```python
from build123d import *

# Parameters (mm, degrees)
SKETCH1_W           = 100
SKETCH1_H           = 6
BOSS_EXTRUDE1_DEPTH = 5
SKETCH2_W           = 100
SKETCH2_H           = 4.1675
CUT_EXTRUDE1_DEPTH  = 4
CUT_EXTRUDE2_DEPTH  = 20


with BuildPart() as part:
    # Sketch1 → Boss-Extrude1 (new body)
    with BuildSketch(Plane(origin=(0, 0, 0), x_dir=(1, 0, 0), z_dir=(0, 1, 0))):
        Rectangle(SKETCH1_W, SKETCH1_H)
    extrude(amount=BOSS_EXTRUDE1_DEPTH)

    # Sketch2 → Cut-Extrude1 (cut)
    with BuildSketch(Plane(origin=(0, 5, 0), x_dir=(1, 0, 0), z_dir=(0, 1, 0))):
        Rectangle(SKETCH2_W, SKETCH2_H)
    extrude(amount=-CUT_EXTRUDE1_DEPTH, mode=Mode.SUBTRACT)

    # Sketch3 → Cut-Extrude2 (cut)
    with BuildSketch(Plane.XY.offset(3)):
        Polygon((50, 0), (41.339745962, 5), (50, 5), align=None)
    extrude(amount=-CUT_EXTRUDE2_DEPTH, mode=Mode.SUBTRACT)


solid = part.part
```
Geometry check sheet. Reference: the model listing, model coordinates, mm. A direction names the side the tool comes from. Round coordinates to 2 decimals unless told otherwise and drop trailing zeros. Loops run counter-clockwise (first coordinate to the right, second up) from the corner with the lowest first, then second, coordinate; pieces in that order, holes last. Notation, with made-up numbers: (82, 55) - (119, 55) arc R14 ccw to (119, 73) - close; hole circle Ø10 at (11.25, 29.5). An arc over 180 degrees is marked (long way). Write item = value, one per line. Start each with the question number.
1. Thickness scan on line 1 (Z direction, x = -28, y = 2.5); line 2 (Y direction, x = -38, z = -0.1); line 3 (X direction, y = 0.5, z = -1.65). Record the ranges inside material, lowest first.
2. Section check C-C on z = -0.15. Enter the section's corners in (x, y), then the cut area to 3 significant figures.
3. Section check B-B on x = 33. Enter the section's corners in (y, z), then the cut area to 3 significant figures.
4. Set-up check for faces 1 (the face through (-2, 1, 0)), 2 (the face through (48.617, 0.798, 0.042)): record each of +Z, -Z, +X, -X, +Y, -Y from which the full face is reachable in a straight line by a thin tool's end or side.
5. Depth check by flat-ended pin: pin 1 (1 mm diameter, centred on y = 3.5, z = 1, fed in from +X); pin 2 (3 mm diameter, centred on x = 11, z = 0.5, fed in from +Y); pin 3 (3 mm diameter, centred on y = 4, z = -2, fed in from +X). Enter the tip coordinate at first touch or a pass-through.
6. Mould release check, pull along Z, two halves, no side actions. Record for faces 3 (the face through (-1, 2, 3)), 4 (the face through (-1, 2, -3)), 5 (the face through (-2, 3, 2.084)): released by +Z, released by -Z, zero draft, split by the parting line, or undercut.
7. Section check A-A on y = 3.25. Enter the section's corners in (x, z).
Working result:
q1.line_1 = -3 to -2.08, 2.08 to 3
q1.line_2 = 0 to 1
q1.line_3 = -50 to 49.13
q2.outline = (-50, 0) - (50, 0) - (48.27, 1) - (-50, 1) - close
q2.area = 99.1 mm^2
q3.outline = (0, -3) - (5, -3) - (5, -2.08) - (1, -2.08) - (1, 2.08) - (5, 2.08) - (5, 3) - (0, 3) - close
q3.area = 13.3 mm^2
q4.face_1 = +X, -X, +Y
q4.face_2 = +Z, -Z, +X, +Y
q5.pin_1 = through
q5.pin_2 = 1
q5.pin_3 = 45.67
q6.face_3 = released by +Z
q6.face_4 = released by -Z
q6.face_5 = undercut
q7.outline = (-50, -3) - (44.37, -3) - (44.37, -2.08) - (-50, -2.08) - close; (-50, 2.08) - (44.37, 2.08) - (44.37, 3) - (-50, 3) - close
